from build123d import *

# Parameters (mm, degrees)
SKETCH1_R               = 20
SKETCH1_R_2             = 16
BOSS_EXTRUDE1_DEPTH     = 100
SKETCH2_W               = 3
SKETCH2_H               = 40
BOSS_EXTRUDE11_DEPTH    = 2
SKETCH3_W               = 3
SKETCH3_H               = 40
BOSS_EXTRUDE12_DEPTH    = 2
BOSS_EXTRUDE13_DEPTH    = 3
FILLET1_R               = 1
SKETCH5_W               = 400
SKETCH5_H               = 100
BOSS_EXTRUDE14_DEPTH    = 20
FILLET2_R               = 2
CUT_EXTRUDE1_DEPTH      = 1
CUT_EXTRUDE1_DEPTH_BACK = 618.662204829
CUT_EXTRUDE2_DEPTH      = 1
CUT_EXTRUDE2_DEPTH_BACK = 618.662204829
CUT_EXTRUDE3_DEPTH      = 21
CUT_EXTRUDE4_DEPTH      = 21
SKETCH11_R              = 7
CUT_EXTRUDE5_DEPTH      = 64
CUT_EXTRUDE5_DEPTH_BACK = 38


with BuildPart() as part:
    # Sketch1 → Boss-Extrude1 (new body)
    with BuildSketch(Plane(origin=(0, 0, 0), x_dir=(1, 0, 0), z_dir=(0, 1, 0))):
        Circle(SKETCH1_R)
        Circle(SKETCH1_R_2, mode=Mode.SUBTRACT)
    extrude(amount=BOSS_EXTRUDE1_DEPTH)

    # Sketch2 → Boss-Extrude11 (add)
    with BuildSketch(Plane(origin=(20, 0, 0), x_dir=(0, 0, -1), z_dir=(1, 0, 0))):
        with Locations((0, 50)):
            Rectangle(SKETCH2_W, SKETCH2_H)
    extrude(amount=-BOSS_EXTRUDE11_DEPTH)

    # Sketch3 → Boss-Extrude12 (add)
    with BuildSketch(Plane(origin=(20, 0, 0), x_dir=(0, 0, -1), z_dir=(1, 0, 0))):
        with Locations((0, 50)):
            Rectangle(SKETCH3_W, SKETCH3_H)
    extrude(amount=BOSS_EXTRUDE12_DEPTH)

    # Sketch4 → Boss-Extrude13 (add)
    with BuildSketch(Plane.XY.offset(1.5)):
        Polygon((22, 70), (254.788125099, -93), (197.662204829, -93), (22, 30), align=None)
    extrude(amount=-BOSS_EXTRUDE13_DEPTH)

    # Fillet1
    fillet1_edges = [part.edges().sort_by_distance(p)[0] for p in [
        (22, 70, 0),
        (138.394062549, -11.5, -1.5),
        (254.788125099, -93, 0),
        (109.831102415, -31.5, -1.5),
        (109.831102415, -31.5, 1.5),
        (138.394062549, -11.5, 1.5),
    ]]
    fillet(fillet1_edges, radius=FILLET1_R)

    # Sketch5 → Boss-Extrude14 (add)
    with BuildSketch(Plane.XZ.offset(93)):
        with Locations((397.662204829, 0)):
            Rectangle(SKETCH5_W, SKETCH5_H)
    extrude(amount=-BOSS_EXTRUDE14_DEPTH)

    # Fillet2
    fillet2_edges = [part.edges().sort_by_distance(p)[0] for p in [
        (197.662204829, -73, -25.75),
        (197.662204829, -83, -50),
        (397.662204829, -73, 50),
        (197.662204829, -83, 50),
        (597.662204829, -73, 0),
        (597.662204829, -83, 50),
        (397.662204829, -73, -50),
        (597.662204829, -83, -50),
        (197.662204829, -73, 25.75),
        (397.662204829, -93, -50),
        (597.662204829, -93, 0),
        (397.662204829, -93, 50),
    ]]
    fillet(fillet2_edges, radius=FILLET2_R)

    # Sketch6 → Cut-Extrude1 (cut, two sides)
    with BuildSketch(Plane(origin=(597.662204829, 0, 0), x_dir=(0, 0, -1), z_dir=(1, 0, 0))) as cut_extrude1_sk:
        Polygon((-52, -81), (-42, -71), (-52, -71), align=None)
    extrude(amount=CUT_EXTRUDE1_DEPTH, mode=Mode.SUBTRACT)
    extrude(cut_extrude1_sk.sketch, amount=-CUT_EXTRUDE1_DEPTH_BACK, mode=Mode.SUBTRACT)

    # Sketch7 → Cut-Extrude2 (cut, two sides)
    with BuildSketch(Plane(origin=(597.662204829, 0, 0), x_dir=(0, 0, -1), z_dir=(1, 0, 0))) as cut_extrude2_sk:
        Polygon((42, -71), (52, -81), (52, -71), align=None)
    extrude(amount=CUT_EXTRUDE2_DEPTH, mode=Mode.SUBTRACT)
    extrude(cut_extrude2_sk.sketch, amount=-CUT_EXTRUDE2_DEPTH_BACK, mode=Mode.SUBTRACT)

    # Sketch8 → Cut-Extrude3 (cut, through all)
    with BuildSketch(Plane(origin=(0, -73, 0), x_dir=(1, 0, 0), z_dir=(0, 1, 0))):
        with BuildLine():
            Line((537.662204829, 13), (597.662204829, 13))
            Line((597.662204829, 13), (597.662204829, -13))
            Line((597.662204829, -13), (537.662204829, -13))
            ThreePointArc((537.662204829, -13), (524.662204829, 0), (537.662204829, 13))
        make_face()
    extrude(amount=-CUT_EXTRUDE3_DEPTH, mode=Mode.SUBTRACT)

    # Sketch9 → Cut-Extrude4 (cut, through all)
    with BuildSketch(Plane(origin=(0, -73, 0), x_dir=(1, 0, 0), z_dir=(0, 1, 0))):
        Polygon((527.662204829, 50), (597.662204829, 50), (597.662204829, 29.5), align=None)
    cut_extrude4 = extrude(amount=-CUT_EXTRUDE4_DEPTH, mode=Mode.SUBTRACT)

    # Mirror1: Cut-Extrude4 across plane
    add(cut_extrude4.mirror(Plane.XY), mode=Mode.SUBTRACT)

    # Sketch11 → Cut-Extrude5 (cut, two sides)
    with BuildSketch(Plane.XY.offset(-13)) as cut_extrude5_sk:
        with Locations((572.662204829, -83)):
            Circle(SKETCH11_R)
    extrude(amount=CUT_EXTRUDE5_DEPTH, mode=Mode.SUBTRACT)
    extrude(cut_extrude5_sk.sketch, amount=-CUT_EXTRUDE5_DEPTH_BACK, mode=Mode.SUBTRACT)


solid = part.part
For this review, take the finished solid that the model builds, in its own axes (mm). A direction names the side the tool comes from. Give positions to 0.01 mm unless a question says otherwise; leave off trailing zeros. Order: outer loops, then holes, each group sorted by start corner. A loop starts at its lowest first (then second) coordinate and runs counter-clockwise, first axis right, second up. Notation, with made-up numbers: M -8.75,65 L 15.25,65 A23 cw 15.25,104 Z; hole C 39.25,13 d11. An arc over 180 degrees is marked long. Answer in a Markdown table with one row per item. Add a question column.
(1) Mouldability with a two-part tool opening along Z and no side actions: class faces 6 (the face through (124.8, -2.33, 1.2)), 7 (the face through (-8.98, 0, -13.43)), 8 (the face through (524.665, -82.86, 0.286)) as +Z half, -Z half, draft (parallel to the pull), parting line (faces both ways), or undercut.
(2) Consider section B-B on x = 511.5. State the section outline as (y, z) points, and give its area (3 significant figures).
(3) For pin 1 (16 mm diameter, centred on x = 577.5, y = -81, fed in from -Z); pin 2 (10 mm diameter, centred on x = 581, y = -79.5, fed in from +Z); pin 3 (20 mm diameter, centred on x = -8.5, z = 9, fed in from -Y), all flat-tipped, find the tip position at first contact; note any pin that passes through.
(4) For faces 1 (the face through (561, -83, 13)), 2 (the face through (-3.47, 49.3, 15.62)), 3 (the face through (108.774, -30.393, -1.215)), 4 (the face through (-8.98, 100, -13.43)), 5 (the face through (111.06, -32.36, 0.01)), list the 3-axis set-ups (+Z, -Z, +X, -X, +Y, -Y) from which the entire face can be reached by the end or side of a thin tool; tool diameter is ignored.
(5) Wall thickness on probe 1 along X at (y, z) = (71.5, 0); probe 2 along X at (y, z) = (-83, -25): over which ranges is each line inside the solid? List them lowest first. Write a range as [from, to].
(6) Consider section A-A on x = 0. State the section outline as (y, z) points, and give its area (3 significant figures).
Evaluation:
| question | item | result |
|---|---|---|
| 1 | face 6 | +Z half |
| 1 | face 7 | draft |
| 1 | face 8 | undercut |
| 2 | outline | M -93,-48 A2 ccw -91,-50 L -79,-50 L -73,-44 L -73,44 L -79,50 L -91,50 A2 ccw -93,48 Z |
| 2 | area | 1,960 mm^2 |
| 3 | pin 1 | stops at z = -37.27 |
| 3 | pin 2 | stops at z = 35.68 |
| 3 | pin 3 | stops at y = 0 |
| 4 | face 1 | +X, +Y, -Y |
| 4 | face 2 | +Y, -Y |
| 4 | face 3 | -Z, -Y |
| 4 | face 4 | +Z, -Z, +X, -X, +Y |
| 4 | face 5 | +Z, -Z, -Y |
| 5 | probe 1 | x = [-20, -16], [16, 20] |
| 5 | probe 2 | x = [197.66, 565.66], [579.66, 597.66] |
| 6 | outline | M 0,-20 L 100,-20 L 100,-16 L 0,-16 Z; M 0,16 L 100,16 L 100,20 L 0,20 Z |
| 6 | area | 800 mm^2 |
